Can you work these out from the model? Positions are in its coordinate system, mm. A direction names the side the tool comes from. Give positions to 0.01 mm unless a question says otherwise; leave off trailing zeros. Order: outer loops, then holes, each group sorted by start corner. A loop starts at its lowest first (then second) coordinate and runs counter-clockwise, first axis right, second up. Notation, with made-up numbers: (-28.5, 4) -> (21.5, 4) arc R30 cw to (21.5, 33) -> close; hole circle Ø4 at (-14.75, 49.25). An arc over 180 degrees is marked (long way). Answer as CSV lines item,"result".
```python
from build123d import *

# Parameters (mm, degrees)
BOSS_EXTRUDE1_DEPTH = 10
BOSS_EXTRUDE6_DEPTH = 41
CUT_EXTRUDE1_REACH  = 81.124
SKETCH6_R           = 9.5
SKETCH6_W           = 9.5
SKETCH6_H           = 18.644559606
CUT_EXTRUDE2_REACH  = 81.124
BOSS_EXTRUDE9_DEPTH = 10
CHAMFER2_SIZE       = 5
CHAMFER2_SIZE_2     = 10
CHAMFER3_SIZE       = 10


# Some blends are built 0.0001 mm under size
with BuildPart() as part:
    # Sketch2 → Boss-Extrude1 (new body)
    with BuildSketch(Plane.XY):
        Polygon((-5, -51.344559606), (-5, -0.20517252), (44.083730464, 1.808954014), (44.083730464, -19.205040291), (14.477900916, -51.344559606), align=None)
    extrude(amount=BOSS_EXTRUDE1_DEPTH)

    # Sketch2<5> → Boss-Extrude6 (add)
    with BuildSketch(Plane.XY):
        Polygon((-5, -0.20517252), (-5, -51.344559606), (14.477900916, -51.344559606), (19.083730464, -46.344559606), (0, -46.344559606), (0, 0), align=None)
    extrude(amount=-BOSS_EXTRUDE6_DEPTH)

    # Sketch6 → Cut-Extrude1 (cut, up to next)
    with BuildSketch(Plane(origin=(0, 0, 0), x_dir=(0, 0, -1), z_dir=(1, 0, 0)), mode=Mode.PRIVATE) as cut_extrude1_sk1:
        with Locations((41, -34.344559606)):
            Circle(SKETCH6_R)
    cut_extrude1_tool1 = extrude(cut_extrude1_sk1.sketch, amount=-CUT_EXTRUDE1_REACH, mode=Mode.PRIVATE) & part.part
    # Sketch6 → Cut-Extrude1 (cut, up to next)
    with BuildSketch(Plane(origin=(0, 0, 0), x_dir=(0, 0, -1), z_dir=(1, 0, 0)), mode=Mode.PRIVATE) as cut_extrude1_sk2:
        with Locations((36.25, -9.322279803)):
            Rectangle(SKETCH6_W, SKETCH6_H)
    cut_extrude1_tool2 = extrude(cut_extrude1_sk2.sketch, amount=-CUT_EXTRUDE1_REACH, mode=Mode.PRIVATE) & part.part
    add(cut_extrude1_tool1.solids().sort_by_distance((0, -34.34456, -41))[0], mode=Mode.SUBTRACT)
    add(cut_extrude1_tool2.solids().sort_by_distance((0, -9.32228, -36.25))[0], mode=Mode.SUBTRACT)

    # Sketch7 → Cut-Extrude2 (cut, up to next)
    with BuildSketch(Plane(origin=(0, 0, 0), x_dir=(-1, 0, 0), z_dir=(0, 0, -1)), mode=Mode.PRIVATE) as cut_extrude2_sk1:
        Polygon((-39.083730464, -17.253097249), (-16.891496625, -41.344559606), (-5, -41.344559606), (-5, -4.799035286), (-39.083730464, -3.400426311), align=None)
    cut_extrude2_tool1 = extrude(cut_extrude2_sk1.sketch, amount=-CUT_EXTRUDE2_REACH, mode=Mode.PRIVATE) & part.part
    add(cut_extrude2_tool1.solids().sort_by_distance((19.604261, -19.893914, 0))[0], mode=Mode.SUBTRACT)

    # Sketch10 → Boss-Extrude9 (add)
    with BuildSketch(Plane.XY.offset(-29)):
        Polygon((19.083730464, -46.344559606), (0, -46.344559606), (0, 0), (5, 0.20517252), (5, -36.344559606), (19.083730464, -36.344559606), align=None)
    extrude(amount=BOSS_EXTRUDE9_DEPTH)

    # Chamfer2
    # the kernel refuses this chamfer: 10, 5 mm, written as the material it takes off along each edge
    with BuildSketch(Plane(origin=(5, 26.103461258, -19), x_dir=(-0.9976223042390326, 0, 0.0689183436017091), z_dir=(0, -1, 0))) as chamfer2_piece_1:
        Polygon((CHAMFER2_SIZE * 0.997622304239, CHAMFER2_SIZE * 0.0689183436017), (-CHAMFER2_SIZE_2 * 0.0689183436017, CHAMFER2_SIZE_2 * 0.997622304239), (0, 0), align=None)
    extrude(amount=62.448020863, mode=Mode.SUBTRACT)

    # Chamfer3
    chamfer3_edges = [part.edges().sort_by_distance(p)[0] for p in [
        (9.541865232, -36.344559606, -19),
    ]]
    chamfer(chamfer3_edges, length=CHAMFER3_SIZE - 0.0001)  # a hair under: the kernel refuses the full size


solid = part.part
```
Item 1: For faces 5 (the flat face through (3, -33, -29)), 6 (the flat face through (-2, -9, -31.5)), 7 (the flat face through (11, -41.345, 5)), 8 (the flat face through (19.084, -42, -25)), 9 (the flat face through (11.529, -41.415, -23.93)), which set-ups out of +Z, -Z, +X, -X, +Y, -Y let a thin tool reach every point of the face, with its end or its side?
Numbers:
face 5,"-Z, +X, +Y"
face 6,"-Z, +X, -X, +Y"
face 7,"+Z"
face 8,"-Z, +X, +Y, -Y"
face 9,"+X, +Y"
Item 2: Imagine slicing it at C-C, the plane z = -37. Please give me the cut outline in (x, y), then the cut area to 3 significant figures.
Numbers:
outline,"(-5, -51.34) -> (14.48, -51.34) -> (19.08, -46.34) -> (0, -46.34) -> (0, -42.96) -> (-5, -42.96) -> close; (-5, -25.73) -> (0, -25.73) -> (0, -18.64) -> (-5, -18.64) -> close"
area,"161 mm²"
Item 3: For pin 1 (1 mm diameter, centred on y = -16, z = -6, fed in from +X); pin 2 (3 mm diameter, centred on x = 4, y = -23, fed in from -Z); pin 3 (21 mm diameter, centred on x = 11.5, z = -5.5, fed in from +Y), each with a flat end and sliding along its axis, tell me the tip position at first contact or that it passes through.
Numbers:
pin 1,"stops at x = 0"
pin 2,"stops at z = -29"
pin 3,"stops at y = 0.84"
Item 4: Imagine slicing it at D-D, the plane z = -17. Please give me the cut outline in (x, y), then the cut area to 3 significant figures.
Numbers:
outline,"(-5, -51.34) -> (14.48, -51.34) -> (19.08, -46.34) -> (0, -46.34) -> (0, 0) -> (-5, -0.21) -> close"
area,"340 mm²"
Item 5: Please list where these lines run through material, in increasing order: line 1 along Y through (x, z) = (33, 1); line 2 along X through (y, z) = (-41.5, -15.5); line 3 along X through (y, z) = (-32.5, 5.5).
Numbers:
line 1,"y = -31.24 to -23.86, -3.65 to 1.35"
line 2,"x = -5 to 0"
line 3,"x = -5 to 5, 25.04 to 31.84"
Item 6: Imagine slicing it at A-A, the plane y = -7. Please give me the cut outline in (x, z).
Numbers:
outline,"(-5, -31.5) -> (0, -31.5) -> (0, -29) -> (5, -29) -> (0, -19) -> (0, 0) -> (5, 0) -> (5, 10) -> (-5, 10) -> close; (39.08, 0) -> (44.08, 0) -> (44.08, 10) -> (39.08, 10) -> close"
Item 7: We'd pull the mould along Y, two halves only. Please class faces 1 (the flat face through (21.8, -4.11, 4.93)), 2 (the flat face through (28.143, -29.13, 4.93)), 3 (the flat face through (2.465, -22.744, -23.93)), 4 (the flat face through (10, -46.345, -35)): released by +Y, released by -Y, zero draft, split by the parting line, or undercut.
Numbers:
face 1,"undercut"
face 2,"undercut"
face 3,"zero draft"
face 4,"released by +Y"
